from build123d import *

# Parameters (mm, degrees)
BOSS_EXTRUDE1_DEPTH = 91.44


with BuildPart() as part:
    # Sketch1 → Boss-Extrude1 (new body)
    with BuildSketch(Plane(origin=(0, 0, 0), x_dir=(0, 0, -1), z_dir=(1, 0, 0))):
        Polygon((7.332348419, 0), (3.666174209, 6.35), (-3.666174209, 6.35), (-7.332348419, 0), (-3.666174209, -6.35), (3.666174209, -6.35), align=None)
    extrude(amount=BOSS_EXTRUDE1_DEPTH)

    # Sketch3 → Tap Drill for 1/4-20 Tap1 (revolve, cut)
    with BuildSketch(Plane.ZX):
        Polygon((0, 0), (0, 14.233816902), (2.5527, 12.7), (2.5527, 0), align=None)
    tap_drill_for_1_4_20_tap1 = revolve(axis=Axis((-6.35, 0, 0), (1, 0, 0)), mode=Mode.SUBTRACT)

    # Mirror1: Tap Drill for 1/4-20 Tap1 across plane
    add(tap_drill_for_1_4_20_tap1.mirror(Plane.ZY.offset(-45.72)), mode=Mode.SUBTRACT)


solid = part.part
CAD build for the part. Positions are in the model's coordinates, mm. A direction names the side the tool comes from. Give positions to 0.01 mm unless a question says otherwise; leave off trailing zeros. Order: outer loops, then holes, each group sorted by start corner. A loop starts at its lowest first (then second) coordinate and runs counter-clockwise, first axis right, second up. Notation, with made-up numbers: (80.5, 50) - (119.5, 50) arc R24 cw to (119.5, 63) - close; hole circle Ø5 at (14, 69.25). An arc over 180 degrees is marked (long way). Answer in a Markdown table with one row per item.
1. Saw through at D-D, the plane y = -4.5. Give the cut face in (x, z).
Data:
| item | result |
|---|---|
| outline | (0, -4.73) - (91.44, -4.73) - (91.44, 4.73) - (0, 4.73) - close |
2. Saw through at C-C, the plane z = 4.75. Give the cut face in (x, y).
Data:
| item | result |
|---|---|
| outline | (0, -4.47) - (91.44, -4.47) - (91.44, 4.47) - (0, 4.47) - close |
3. Saw through at B-B, the plane x = 51. Give the cut face in (y, z), plus the area to 3 significant figures.
Data:
| item | result |
|---|---|
| outline | (-6.35, -3.67) - (0, -7.33) - (6.35, -3.67) - (6.35, 3.67) - (0, 7.33) - (-6.35, 3.67) - close |
| area | 140 mm² |
4. Flat gauge pins, fed straight in: pin 1 (4 mm diameter, centred on y = 0, z = -6, fed in from -X); pin 2 (2 mm diameter, centred on x = 54.5, y = -2, fed in from -Z) (3 decimals); pin 3 (4.5 mm diameter, centred on y = 0, z = 0, fed in from -X); pin 4 (3 mm diameter, centred on y = 0, z = 0, fed in from +X). Where does each tip first touch, or does it go through?
Data:
| item | result |
|---|---|
| pin 1 | stops at x = 0 |
| pin 2 | stops at z = -6.755 |
| pin 3 | stops at x = 12.88 |
| pin 4 | stops at x = 78.11 |
5. Tool access for faces 1 (the cylindrical face through (85.179, -0.767, 2.435)), 2 (the flat face through (45.08, -3.219, -5.474)), 3 (the cylindrical face through (6.261, -0.767, 2.435)): list every direction of +Z, -Z, +X, -X, +Y, -Y with a clear straight run to the whole face (end or side of a thin tool).
Data:
| item | result |
|---|---|
| face 1 | +X |
| face 2 | -Z, +X, -X, -Y |
| face 3 | -X |
6. Saw through at A-A, the plane x = 8. Give the cut face in (y, z).
Data:
| item | result |
|---|---|
| outline | (-6.35, -3.67) - (0, -7.33) - (6.35, -3.67) - (6.35, 3.67) - (0, 7.33) - (-6.35, 3.67) - close; hole circle Ø5.11 at (0, 0) |
7. Pull direction Z, two halves, no side cores. Call faces 4 (the conical face through (13.97, 0.43, -0.1)), 5 (the conical face through (77.47, 0.43, -0.1)), 6 (the flat face through (45.08, -3.131, 5.525)), 7 (the flat face through (91.44, 0, -3)): pulls with the +Z half, pulls with the -Z half, needs draft (parallel to the pull), parting line crosses it, or undercut.
Data:
| item | result |
|---|---|
| face 4 | undercut |
| face 5 | undercut |
| face 6 | pulls with the +Z half |
| face 7 | needs draft |
8. Probe probe 1 along Z at (x, y) = (88.25, 0); probe 2 along Y at (x, z) = (88, 0); probe 3 along Z at (x, y) = (12.5, 1) (3 decimals). List the from-to ranges inside material, lowest first. Write a range as [from, to].
Data:
| item | result |
|---|---|
| probe 1 | z = [-7.33, -2.55], [2.55, 7.33] |
| probe 2 | y = [-6.35, -2.55], [2.55, 6.35] |
| probe 3 | z = [-6.755, -2.349], [2.349, 6.755] |
